from build123d import *

# Parameters (mm, degrees)
F0_W     = 6.35
F0_H     = 25.4
F1_DEPTH = 45.72
F2_R     = 3.062636224
F3_DEPTH = 25.4
F5_DEPTH = 0.762
F6_DEPTH = 25.4
F7_R     = 3.429
F8_DEPTH = 25.4


with BuildPart() as f1:
    # F0 (on Top) → F1 (new body)
    with BuildSketch(Plane.XY):
        with Locations((3.175, -12.7)):
            Rectangle(F0_W, F0_H)
    extrude(amount=F1_DEPTH)

    # F2 (on face) → F3 (cut)
    with BuildSketch(Plane(origin=(0, 0, 0), x_dir=(0, -1, 0), z_dir=(-1, 0, 0))):
        with Locations((12.7, 35.052)):
            Circle(F2_R)
    extrude(amount=-F3_DEPTH, mode=Mode.SUBTRACT)

    # F0 (on Top) → F5 (join)
    with BuildSketch(Plane.XY):
        with Locations((3.175, -12.7)):
            Rectangle(F0_W, F0_H)
        Polygon((62.9475070931, -15.24), (6.35, 0), (6.35, -25.4), (62.9475070931, -25.4), align=None)
    extrude(amount=F5_DEPTH)

    # F4 (on face) → F6 (cut)
    with BuildSketch(Plane(origin=(0, 0, 0), x_dir=(0, -1, 0), z_dir=(-1, 0, 0))):
        with BuildLine():
            ThreePointArc((0, 35.052), (4.4069875196, 42.6991100957), (12.7, 45.72))
            Line((12.7, 45.72), (0, 45.72))
            Line((0, 45.72), (0, 35.052))
        make_face()
        with BuildLine():
            ThreePointArc((12.7, 45.72), (20.9930124804, 42.6991100957), (25.4, 35.052))
            Line((25.4, 35.052), (25.4, 45.72))
            Line((25.4, 45.72), (12.7, 45.72))
        make_face()
    extrude(amount=-F6_DEPTH, mode=Mode.SUBTRACT)

    # F7 (on face) → F8 (cut)
    with BuildSketch(Plane.XY.offset(0.762)):
        with Locations((12.7, -17.78)):
            Circle(F7_R)
        with Locations((35.56, -17.78)):
            Circle(F7_R)
    extrude(amount=-F8_DEPTH, mode=Mode.SUBTRACT)


solid = f1.part
Build history of the part. All positions in model axes, mm. A direction names the side the tool comes from. Give positions to 0.01 mm unless a question says otherwise; leave off trailing zeros. Loops run counter-clockwise (first coordinate to the right, second up) from the corner with the lowest first, then second, coordinate; pieces in that order, holes last. Notation, with made-up numbers: (-4.75, 13) - (24.25, 13) arc R32 ccw to (24.25, 43) - close; hole circle Ø1 at (17.5, 49). An arc over 180 degrees is marked (long way). Write item = value, one per line. Start each with the question number.
1) Band-saw the part on C-C on y = -17. Give the cut face in (x, z).
2) Drop flat-ended pins along their axis: pin 1 Ø7.5 at (y, z) = (-13.5, 34) entering from +X; pin 2 Ø12.5 at (x, y) = (27, -15) entering from +Z; pin 3 Ø4 at (x, y) = (12.7, -17.78) entering from -Z. Give the stop position or say it passes through.
3) Probe probe 1 along Z at (x, y) = (50, -12.5); probe 2 along X at (y, z) = (-11.25, 44); probe 3 along Y at (x, z) = (12.7, 0.2). List the from-to ranges inside material, lowest first. Write a range as from..to.
4) Band-saw the part on D-D on y = -23. Give the cut face in (x, z), plus the area to 3 significant figures.
5) Band-saw the part on A-A on x = 12.5. Give the cut face in (y, z).
6) Pull direction Z, two halves, no side cores. Call faces 1 (the cylindrical face through (12.25, -14.38, 0.39)), 2 (the flat face through (28, -15, 0.762)), 3 (the cylindrical face through (3.13, -12.04, 32.06)), 4 (the flat face through (24, -15, 0)): +Z half, -Z half, draft (parallel to the pull), parting line (faces both ways), or undercut.
7) Band-saw the part on B-B on z = 33. Give the cut face in (x, y).
8) Tool access for faces 5 (the flat face through (6.35, -13, 23)), 6 (the flat face through (6, -25.4, 14)): list every direction of +Z, -Z, +X, -X, +Y, -Y with a clear straight run to the whole face (end or side of a thin tool).
Final values:
q1.outline = (0, 0) - (9.36, 0) - (9.36, 0.76) - (6.35, 0.76) - (6.35, 44.98) - (0, 44.98) - close; (16.04, 0) - (32.22, 0) - (32.22, 0.76) - (16.04, 0.76) - close; (38.9, 0) - (62.95, 0) - (62.95, 0.76) - (38.9, 0.76) - close
q2.pin_1 = 6.35
q2.pin_2 = 0.76
q2.pin_3 = through
q3.probe_1 = 0..0.76
q3.probe_2 = 0..6.35
q3.probe_3 = -25.4..-21.21, -14.35..-1.71
q4.outline = (0, 0) - (62.95, 0) - (62.95, 0.76) - (6.35, 0.76) - (6.35, 40.58) - (0, 40.58) - close
q4.area = 301 mm²
q5.outline = (-25.4, 0) - (-21.2, 0) - (-21.2, 0.76) - (-25.4, 0.76) - close; (-14.36, 0) - (-1.66, 0) - (-1.66, 0.76) - (-14.36, 0.76) - close
q6.face_1 = draft
q6.face_2 = +Z half
q6.face_3 = undercut
q6.face_4 = -Z half
q7.outline = (0, -25.4) - (6.35, -25.4) - (6.35, -14.97) - (0, -14.97) - close; (0, -10.43) - (6.35, -10.43) - (6.35, 0) - (0, 0) - close
q8.face_5 = +Z, +X, +Y, -Y
q8.face_6 = +Z, -Z, +X, -X, -Y
